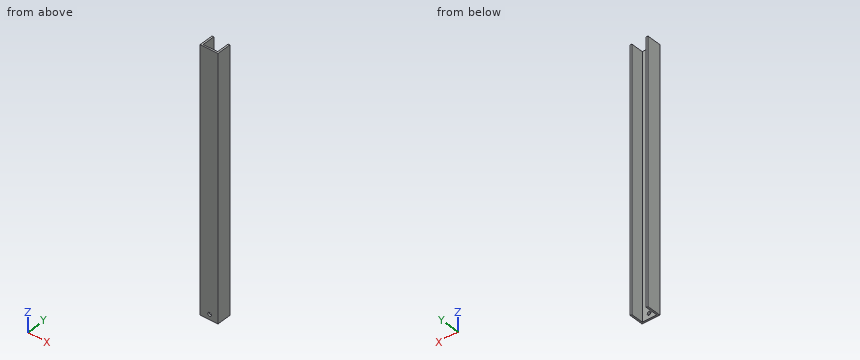
Autodesk Inventor part; units mm, degrees
ref_plane "YZ Plane" through (0, 0, 0) normal (1, 0, 0) x (0, 1, 0)
ref_plane "XZ Plane" through (0, 0, 0) normal (0, 1, 0) x (-1, 0, 0)
ref_plane "XY Plane" through (0, 0, 0) normal (0, 0, 1) x (1, 0, 0)
sketch "Sketch1" plane through (0, 0, 0) normal (0, 0, 1) x (1, 0, 0)
  line L0 (-15.7, 12.7) -> (-12.7, 12.7)
  line L1 (-12.7, 12.7) -> (-12.7, -9.7)
  line L2 (-12.7, -9.7) -> (12.7, -9.7)
  line L3 (12.7, -9.7) -> (12.7, 12.7)
  line L4 (12.7, 12.7) -> (15.7, 12.7)
  line L5 (15.7, 12.7) -> (15.7, -12.7)
  line L6 (15.7, -12.7) -> (-15.7, -12.7)
  line L7 (-15.7, -12.7) -> (-15.7, 12.7)
  point P0 (0, 0)
  dimension "d0" = 3
  dimension "d2" = 3
  dimension "d3" = 25.4
  dimension "d4" = 31.4
  dimension "d5" = 15.7
  dimension "d7" = 12.7
  dimension "d8" = 3
extrude "Extrusion1" add sketch "Sketch1" against normal blind 457.2
sketch "Sketch6" plane through (-15.7, -12.7, 0) normal (0, -1, 0) x (1, 0, 0)
  circle A0 centre (16.6513, -447.9) radius 3.175
  point P0 (15.7, 0)
  dimension "d21" = 6.35
extrude "Extrusion4" cut sketch "Sketch6" against normal blind 10
equation "\"d2\" = d0"
equation "\"d8\" = d0"
properties part number "18in C-Channel"
Work out the finished part from the listing and answer in its coordinate system (mm). Give positions to 0.01 mm unless a question says otherwise; leave off trailing zeros. Write each loop counter-clockwise with the first axis right and the second up, starting at its lowest first coordinate (ties: lowest second). Pieces come first, ordered by that corner, then holes.
(1) The part is cut by section B-B on z = -395. Write down the section's boundary in (x, y), plus the area to 3 significant figures.
Final values:
outline: (-15.7, -12.7) - (15.7, -12.7) - (15.7, 12.7) - (12.7, 12.7) - (12.7, -9.7) - (-12.7, -9.7) - (-12.7, 12.7) - (-15.7, 12.7) - close
area: 229 mm2
(2) Flat-ended cylindrical pins translate along their axes: pin 1 Ø12.5 at (x, z) = (5.5, -122.5) entering from +Y; pin 2 Ø8 at (x, y) = (5.5, 8.5) entering from +Z; pin 3 Ø8 at (x, y) = (9, -6) entering from -Z. Find the tip coordinate at first contact, or state that the pin passes through.
Final values:
pin 1: stops at y = -9.7
pin 2: passes through
pin 3: stops at z = -457.2
(3) The part is cut by section A-A on y = 6. Write down the section's boundary in (x, z), plus the area to 3 significant figures.
Final values:
outline: (-15.7, -457.2) - (-12.7, -457.2) - (-12.7, 0) - (-15.7, 0) - close; (12.7, -457.2) - (15.7, -457.2) - (15.7, 0) - (12.7, 0) - close
area: 2,740 mm2
(4) The part is cut by section C-C on x = -6. Write down the section's boundary in (y, z), plus the area to 3 significant figures.
Final values:
outline: (-12.7, -457.2) - (-9.7, -457.2) - (-9.7, 0) - (-12.7, 0) - close
area: 1,370 mm2
(5) Straight lines are drawn through the part: line 1 (X direction, y = -10.7, z = -447.9); line 2 (X direction, y = 2, z = -438); line 3 (Y direction, x = 0, z = -29.5). For each, find the intervals that lie inside material, in ascending order.
Final values:
line 1: x = -15.7 to -2.22, 4.13 to 15.7
line 2: x = -15.7 to -12.7, 12.7 to 15.7
line 3: y = -12.7 to -9.7
